Design review of the part built by this model. Coordinates are the model's own, in mm. Face numbers are marked on the shaded views. A direction names the side the tool comes from. Round coordinates to 2 decimals unless told otherwise and drop trailing zeros. Loops run counter-clockwise (first coordinate to the right, second up) from the corner with the lowest first, then second, coordinate; pieces in that order, holes last. Notation, with made-up numbers: M 74.5,-15.5 L 92.5,-15.5 A33 cw 92.5,16.5 Z; hole C -10.75,57 d4. An arc over 180 degrees is marked long. Use a Markdown table: item, result.
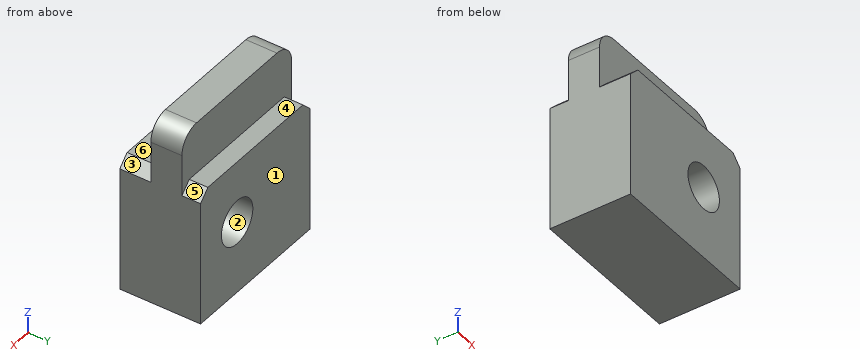
from build123d import *

# Parameters (mm, degrees)
SKETCH167_W         = 15
SKETCH167_H         = 3
PAD068_DEPTH        = 11
SKETCH168_W         = 15
SKETCH168_H         = 16
PAD069_DEPTH        = 3
FILLET078_R         = 2
SKETCH189_W         = 15
SKETCH189_H         = 11
PAD080_DEPTH        = 1.8
SKETCH169_R         = 2.15
POCKET089_DEPTH     = 7.801
CHAMFER024_SIZE     = 1
CHAMFER024_FACE13_W = 7.8
CHAMFER024_FACE13_H = 15
PAD081_DEPTH        = 2


with BuildPart() as part:
    # Sketch167 → Pad068 (new body)
    with BuildSketch(Plane.XY):
        with Locations((7.5, -1.5)):
            Rectangle(SKETCH167_W, SKETCH167_H)
    extrude(amount=-PAD068_DEPTH)

    # Sketch168 (on Face1 of Pad068) → Pad069 (join)
    with BuildSketch(Plane(origin=(0, 0, 0), x_dir=(-1, 0, 0), z_dir=(0, 1, 0))):
        with Locations((-7.5, -3)):
            Rectangle(SKETCH168_W, SKETCH168_H)
    extrude(amount=PAD069_DEPTH)

    # Fillet078
    fillet078_edges = [part.edges().sort_by_distance(p)[0] for p in [
        (0, 1.5, 5),
        (15, 1.5, 5),
    ]]
    fillet(fillet078_edges, radius=FILLET078_R)

    # Sketch189 (on Face8 of Fillet078) → Pad080 (join)
    with BuildSketch(Plane(origin=(0, 3, 0), x_dir=(-1, 0, 0), z_dir=(0, 1, 0))):
        with Locations((-7.5, -5.5)):
            Rectangle(SKETCH189_W, SKETCH189_H)
    extrude(amount=PAD080_DEPTH)

    # Sketch169 → Pocket089 (cut, through all)
    with BuildSketch(Plane.XZ.offset(3)):
        with Locations((10, -6)):
            Circle(SKETCH169_R)
    extrude(amount=-POCKET089_DEPTH, mode=Mode.SUBTRACT)

    # Chamfer024
    chamfer024_edges = [part.edges().sort_by_distance(p)[0] for p in [
        (15, -1.5, 0),
        (15, 3.9, 0),
        (0, 3.9, 0),
        (0, -1.5, 0),
    ]]
    chamfer(chamfer024_edges, length=CHAMFER024_SIZE)

    # Chamfer024 Face13 → Pad081 (add)
    with BuildSketch(Plane(origin=(7.5, 0.9, -11), x_dir=(0, -1, 0), z_dir=(0, 0, -1))):
        Rectangle(CHAMFER024_FACE13_W, CHAMFER024_FACE13_H)
    extrude(amount=PAD081_DEPTH)


with BuildPart() as part_1:
    # Body044 placement: moved
    add(part.part.moved(Location((5, -38, 56))))


solid = part_1.part
1. Take a section at A-A on z = 50. Give the boundary of the cut face in (x, y), and give its area (3 significant figures).
Check values:
| item | result |
|---|---|
| outline | M 5,-41 L 12.85,-41 L 12.85,-33.2 L 5,-33.2 Z; M 17.15,-41 L 20,-41 L 20,-33.2 L 17.15,-33.2 Z |
| area | 83.5 mm² |
2. Take a section at B-B on y = -34.75. Give the boundary of the cut face in (x, z).
Check values:
| item | result |
|---|---|
| outline | M 5,43 L 20,43 L 20,55 L 19,56 L 6,56 L 5,55 Z; hole C 15,50 d4.3 |
3. Take a section at D-D on x = 17.75. Give the boundary of the cut face in (y, z).
Check values:
| item | result |
|---|---|
| outline | M -41,43 L -33.2,43 L -33.2,56 L -35,56 L -35,61 L -38,61 L -38,56 L -41,56 Z |
4. The part is to be moulded in two halves that separate along Z. For the marked faces 1, 2 and 3, say which applies: pulls with the +Z half, pulls with the -Z half, needs draft (parallel to the pull), parting line crosses it, or undercut.
Check values:
| item | result |
|---|---|
| face 1 | needs draft |
| face 2 | undercut |
| face 3 | pulls with the +Z half |
5. Insertion check: pin 1 (5 mm diameter, centred on x = 15.5, z = 57, fed in from +Y); pin 2 (3 mm diameter, centred on x = 9, z = 58.5, fed in from -Y); pin 3 (0.9 mm diameter, centred on x = 11, y = -34.5, fed in from +Z). Each pin has a flat end and moves straight along its axis. Give the tip position at first contact, or say it passes through.
Check values:
| item | result |
|---|---|
| pin 1 | stops at y = -33.2 |
| pin 2 | stops at y = -38 |
| pin 3 | stops at z = 56 |
6. Machinability: for the marked faces 4, 5 and 6, which of the approach directions +Z, -Z, +X, -X, +Y, -Y give a long, thin tool a straight path to every point of the face, cutting with its end or side? Answer none if there is none.
Check values:
| item | result |
|---|---|
| face 4 | +Z, +X, -X, +Y |
| face 5 | +Z, +X, +Y |
| face 6 | +Z, +X, -X, -Y |
7. Wall thickness on line 1 along Z through (x, y) = (15, -39); line 2 along Z through (x, y) = (15, -36); line 3 along X through (y, z) = (-38, 49.5): over which ranges is each line inside the solid? List them lowest first. Write a range as from..to.
Check values:
| item | result |
|---|---|
| line 1 | z = 43..47.85, 52.15..56 |
| line 2 | z = 43..47.85, 52.15..61 |
| line 3 | x = 5..12.91, 17.09..20 |
8. Take a section at C-C on x = 15. Give the boundary of the cut face in (y, z), and give its area (3 significant figures).
Check values:
| item | result |
|---|---|
| outline | M -41,43 L -33.2,43 L -33.2,47.85 L -41,47.85 Z; M -41,52.15 L -33.2,52.15 L -33.2,56 L -35,56 L -35,61 L -38,61 L -38,56 L -41,56 Z |
| area | 82.9 mm² |
